Could you check a few things on this model? Use its own coordinates, in mm. Face numbers are marked on the shaded views. A direction names the side the tool comes from. Give positions to 0.01 mm unless a question says otherwise; leave off trailing zeros. Write each loop counter-clockwise with the first axis right and the second up, starting at its lowest first coordinate (ties: lowest second). Pieces come first, ordered by that corner, then holes. Notation, with made-up numbers: M 64.5,38 L 85.5,38 A26 cw 85.5,57 Z; hole C 35.25,-17.5 d7. An arc over 180 degrees is marked long. Answer as CSV lines item,"result". Start each with the question number.
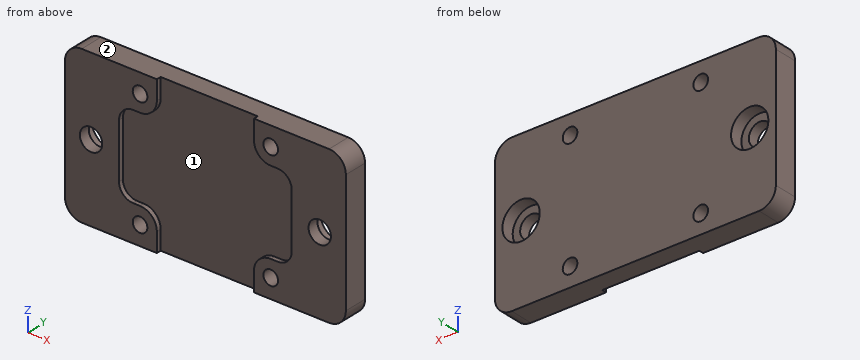
Autodesk Inventor part; units mm, degrees
ref_plane "Work Plane1" through (0, 0, 0) normal (0, -1, 0) x (1, 0, 0)
ref_plane "YZ Plane" through (0, 0, 0) normal (1, 0, 0) x (0, 1, 0)
ref_plane "XZ Plane" through (0, 0, 0) normal (0, 1, 0) x (-1, 0, 0)
ref_plane "Work Plane1" through (0, 0, 0) normal (0, -1, 0) x (1, 0, 0)
sketch "Sketch7" plane through (0, 0, 0) normal (0, 1, 0) x (-1, 0, 0)
  arc A0 (-2, -17) -> (0, -15) centre (-2, -15) ccw
  line L0 (0, -15) -> (0, -2)
  arc A1 (0, -2) -> (-2, 0) centre (-2, -2) ccw
  line L1 (-2, 0) -> (-8.25, 0)
  arc A2 (-6, -2.25) -> (-8.25, 0) centre (-8.25, -2.25) ccw
  line L2 (-6, -14.75) -> (-6, -2.25)
  arc A3 (-8.25, -17) -> (-6, -14.75) centre (-8.25, -14.75) ccw
  line L3 (-8.25, -17) -> (-2, -17)
  line L4 (-22.25, 0) -> (-8.25, 0)
  arc A4 (-22.25, 0) -> (-24.5, -2.25) centre (-22.25, -2.25) ccw
  line L5 (-24.5, -14.75) -> (-24.5, -2.25)
  arc A5 (-24.5, -14.75) -> (-22.25, -17) centre (-22.25, -14.75) ccw
  line L6 (-8.25, -17) -> (-22.25, -17)
  arc A6 (-8.25, -17) -> (-6, -14.75) centre (-8.25, -14.75) ccw
  line L7 (-6, -2.25) -> (-6, -14.75)
  arc A7 (-6, -2.25) -> (-8.25, 0) centre (-8.25, -2.25) ccw
  arc A8 (-28.5, 0) -> (-30.5, -2) centre (-28.5, -2) ccw
  line L8 (-30.5, -2) -> (-30.5, -15)
  arc A9 (-30.5, -15) -> (-28.5, -17) centre (-28.5, -15) ccw
  line L9 (-28.5, -17) -> (-22.25, -17)
  arc A10 (-24.5, -14.75) -> (-22.25, -17) centre (-22.25, -14.75) ccw
  line L10 (-24.5, -2.25) -> (-24.5, -14.75)
  arc A11 (-22.25, 0) -> (-24.5, -2.25) centre (-22.25, -2.25) ccw
  line L11 (-22.25, 0) -> (-28.5, 0)
  line L12 (-23, -4.05) -> (-22.25, -4.05)
  arc A12 (-22.25, -4.05) -> (-20.45, -2.25) centre (-22.25, -2.25) ccw
  line L13 (-20.45, -2.25) -> (-20.45, -1.5)
  arc A13 (-18.95, 0) -> (-20.45, -1.5) centre (-18.95, -1.5) ccw
  line L14 (-18.95, 0) -> (-22.25, 0)
  arc A14 (-22.25, 0) -> (-24.5, -2.25) centre (-22.25, -2.25) ccw
  line L15 (-24.5, -2.25) -> (-24.5, -5.55)
  arc A15 (-23, -4.05) -> (-24.5, -5.55) centre (-23, -5.55) ccw
  circle A16 centre (-22.25, -2.25) radius 0.8
  line L16 (-8.25, -4.05) -> (-7.5, -4.05)
  arc A17 (-6, -5.55) -> (-7.5, -4.05) centre (-7.5, -5.55) ccw
  line L17 (-6, -5.55) -> (-6, -2.25)
  arc A18 (-6, -2.25) -> (-8.25, 0) centre (-8.25, -2.25) ccw
  line L18 (-8.25, 0) -> (-11.55, 0)
  arc A19 (-10.05, -1.5) -> (-11.55, 0) centre (-11.55, -1.5) ccw
  line L19 (-10.05, -1.5) -> (-10.05, -2.25)
  arc A20 (-10.05, -2.25) -> (-8.25, -4.05) centre (-8.25, -2.25) ccw
  circle A21 centre (-8.25, -2.25) radius 0.8
  line L20 (-10.05, -14.75) -> (-10.05, -15.5)
  arc A22 (-11.55, -17) -> (-10.05, -15.5) centre (-11.55, -15.5) ccw
  line L21 (-11.55, -17) -> (-8.25, -17)
  arc A23 (-8.25, -17) -> (-6, -14.75) centre (-8.25, -14.75) ccw
  line L22 (-6, -14.75) -> (-6, -11.45)
  arc A24 (-7.5, -12.95) -> (-6, -11.45) centre (-7.5, -11.45) ccw
  line L23 (-7.5, -12.95) -> (-8.25, -12.95)
  arc A25 (-8.25, -12.95) -> (-10.05, -14.75) centre (-8.25, -14.75) ccw
  circle A26 centre (-8.25, -14.75) radius 0.8
  line L24 (-22.25, -12.95) -> (-23, -12.95)
  arc A27 (-24.5, -11.45) -> (-23, -12.95) centre (-23, -11.45) ccw
  line L25 (-24.5, -11.45) -> (-24.5, -14.75)
  arc A28 (-24.5, -14.75) -> (-22.25, -17) centre (-22.25, -14.75) ccw
  line L26 (-22.25, -17) -> (-18.95, -17)
  arc A29 (-20.45, -15.5) -> (-18.95, -17) centre (-18.95, -15.5) ccw
  line L27 (-20.45, -15.5) -> (-20.45, -14.75)
  arc A30 (-20.45, -14.75) -> (-22.25, -12.95) centre (-22.25, -14.75) ccw
  circle A31 centre (-22.25, -14.75) radius 0.8
  line L28 (-10.05, -1.5) -> (-10.05, 0)
  line L29 (-10.05, -15.5) -> (-10.05, -17)
  line L30 (-20.45, -15.5) -> (-20.45, -17)
  line L31 (-20.45, -1.5) -> (-20.45, 0)
  point P0 (0, 0)
  point P1 (145.09, 90.0262)
  point P2 (-71.3045, 9.3)
  point P3 (-8.25, 0)
  point P4 (-6, -5.55)
extrude "Extrusion5" add sketch "Sketch7" along normal blind 2.52 contours L3 A3 L2 A2 L1 A1 L0 A0 | L6 L29 L20 A25 L23 A24 L2 A3 | L6 A22 L29 | A24 L23 A25 L20 A22 L6 A29 L27 A30 L24 A27 L5 A15 L12 A12 L13 A13 L4 A19 L19 A20 L16 A17 L2 | A2 L2 A17 L16 A20 L19 L28 L4 | L6 L30 A29 | L28 A19 L4 | L6 A5 L5 A27 L24 A30 L27 L30 | L9 A9 L8 A8 L11 A4 L5 A5 | A13 L31 L4 | L31 L13 A12 L12 A15 L5 A4 L4 | A16 | A21 | A26 | A31
extrude "Extrusion6" cut sketch "Sketch7" along normal blind 0.5 contours L6 A22 L29 | A24 L23 A25 L20 A22 L6 A29 L27 A30 L24 A27 L5 A15 L12 A12 L13 A13 L4 A19 L19 A20 L16 A17 L2 | L6 L30 A29 | L28 A19 L4 | A13 L31 L4
sketch "Sketch8" plane through (0, 2.52, 0) normal (0, 1, 0) x (1, 0, 0)
  arc A0 (0, 2) -> (2, 0) centre (2, 2) ccw
  line L0 (2, 0) -> (28.5, 0)
  arc A1 (28.5, 0) -> (30.5, 2) centre (28.5, 2) ccw
  line L1 (30.5, 2) -> (30.5, 15)
  arc A2 (30.5, 15) -> (28.5, 17) centre (28.5, 15) ccw
  line L2 (28.5, 17) -> (2, 17)
  arc A3 (2, 17) -> (0, 15) centre (2, 15) ccw
  line L3 (0, 15) -> (0, 2)
  line L4 (2, 16.8) -> (28.5, 16.8)
  arc A4 (30.3, 15) -> (28.5, 16.8) centre (28.5, 15) ccw
  line L5 (30.3, 15) -> (30.3, 2)
  arc A5 (28.5, 0.2) -> (30.3, 2) centre (28.5, 2) ccw
  line L6 (28.5, 0.2) -> (2, 0.2)
  arc A6 (0.2, 2) -> (2, 0.2) centre (2, 2) ccw
  line L7 (0.2, 2) -> (0.2, 15)
  arc A7 (2, 16.8) -> (0.2, 15) centre (2, 15) ccw
  point P0 (0, 0)
  dimension "d32" = 0.2
extrude "Extrusion7" cut sketch "Sketch8" against normal blind 10
hole "Hole3" at (22.25, 0, -14.75) at (8.25, 0, -14.75) at (8.25, 0, -2.25) at (22.25, 0, -2.25) direction (0, 1, 0) diameter 1.567 depth 3
sketch "Sketch10" plane through (0, 2.52, 0) normal (0, 1, 0) x (1, 0, 0)
  line L0 (24.5, 14.75) -> (24.5, 2.25)
  line L1 (6, 14.75) -> (6, 2.25)
  line L2 (24.5, 5.55) -> (24.5, 11.45)
  line L3 (24.5, 8.5) -> (27.5, 8.5)
  line L4 (6, 11.45) -> (6, 5.55)
  line L5 (6, 8.5) -> (3, 8.5)
  point P0 (0, 0)
  dimension "d42" = 3
  dimension "d43" = 3
hole "Hole4" at (27.5, 2.52, -8.5) at (3, 2.52, -8.5) direction (0, -1, 0) diameter 2.4 depth 3 counterbore diameter 4 counterbore depth 1.35
properties part number "2021-01-011"
1. Imagine slicing it at A-A, the plane z = -8.5. Please give me the cut outline in (x, y), plus the area to 3 significant figures.
2. On a 3-axis mill with a long thin cutter (end or side, diameter ignored), from which of +Z, -Z, +X, -X, +Y, -Y can I reach the whole of each face in a straight line? I mean the marked faces 1 and 2. Say none if no direction works.
3. Will these pins go through, and if not, where does the flat tip stop? P1, Ø1.2, axis at x = 3, z = -8.5, coming from the +Y side; P2, Ø0.6, axis at y = 0, z = -1, coming from the +X side.
4. Imagine slicing it at D-D, the plane z = -6. Please give me the cut outline in (x, y).
5. Imagine slicing it at C-C, the plane y = 1.6. Please give me the cut outline in (x, z).
6. Please list where these lines run through material, in increasing order: line 1 (X direction, y = 1.35, z = -14.75); line 2 (Z direction, x = 8.25, y = 1.15); line 3 (X direction, y = 2.25, z = -8.5).
7. Imagine slicing it at B-B, the plane x = 3. Please give me the cut outline in (y, z), plus the area to 3 significant figures.
Solutions:
1,outline,"M 0.2,0 L 1.8,0 L 1.8,1.17 L 1,1.17 L 1,2.52 L 0.2,2.52 Z; M 4.2,0 L 6,0 L 6,0.5 L 24.5,0.5 L 24.5,0 L 26.3,0 L 26.3,1.17 L 25.5,1.17 L 25.5,2.52 L 5,2.52 L 5,1.17 L 4.2,1.17 Z; M 28.7,0 L 30.3,0 L 30.3,2.52 L 29.5,2.52 L 29.5,1.17 L 28.7,1.17 Z"
1,area,"50.2 mm²"
2,face 1,"-Y"
2,face 2,"+Z, +X, -X, +Y, -Y"
3,P1,"through"
3,P2,"x = 30.16"
4,outline,"M 0.2,0 L 6,0 L 6,0.5 L 24.5,0.5 L 24.5,0 L 30.3,0 L 30.3,2.52 L 0.2,2.52 Z"
5,outline,"M 0.2,-15 A1.8 ccw 2,-16.8 L 28.5,-16.8 A1.8 ccw 30.3,-15 L 30.3,-2 A1.8 ccw 28.5,-0.2 L 2,-0.2 A1.8 ccw 0.2,-2 Z; hole C 3,-8.5 d4; hole C 8.25,-14.75 d1.57; hole C 8.25,-2.25 d1.57; hole C 22.25,-14.75 d1.57; hole C 22.25,-2.25 d1.57; hole C 27.5,-8.5 d4"
6,line 1,"0.2 to 7.47, 9.03 to 21.47, 23.03 to 30.3"
6,line 2,"-16.8 to -15.53, -13.97 to -3.03, -1.47 to -0.2"
6,line 3,"0.2 to 1, 5 to 25.5, 29.5 to 30.3"
7,outline,"M 0,-16.8 L 2.52,-16.8 L 2.52,-10.5 L 1.17,-10.5 L 1.17,-9.7 L 0,-9.7 Z; M 0,-7.3 L 1.17,-7.3 L 1.17,-6.5 L 2.52,-6.5 L 2.52,-0.2 L 0,-0.2 Z"
7,area,"33.6 mm²"
